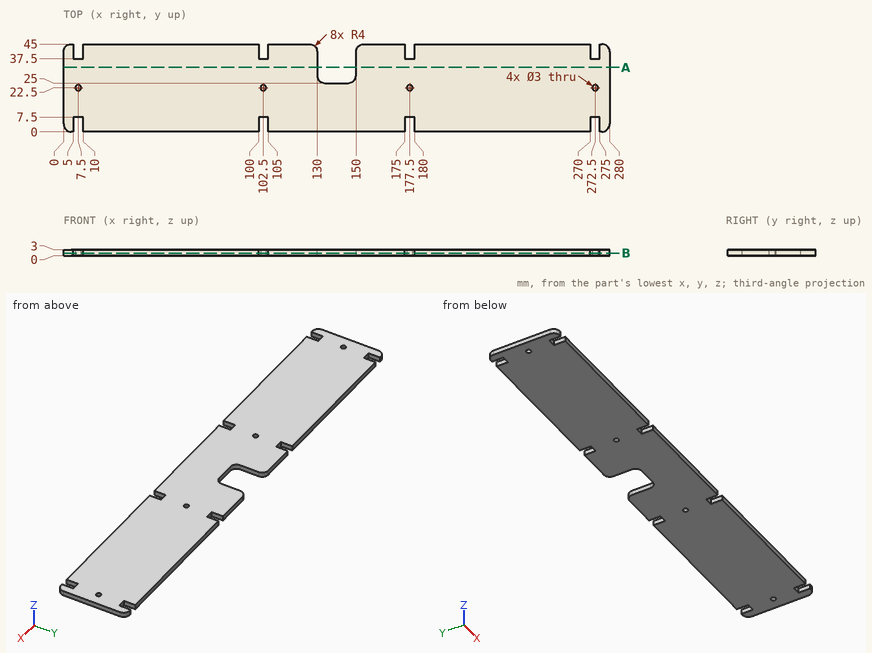
Could you check a few things on this drawing? It's one solid part, dimensions in mm from its lowest x, y, z. Give positions to 0.01 mm unless a question says otherwise; leave off trailing zeros. Loops run counter-clockwise (first coordinate to the right, second up) from the corner with the lowest first, then second, coordinate; pieces in that order, holes last. Notation, with made-up numbers: M 85,35.5 L 141,35.5 A30 cw 141,68.5 Z; hole C -22,-21 d8. An arc over 180 degrees is marked long. One line per question, with ' | ' between items. Start each with the question number.
Q1. If I drill on line 1 (X direction, y = 23.5, z = 0.95); line 2 (X direction, y = 37, z = 2.45); line 3 (Y direction, x = 177.5, z = 1.3), over which ranges is the centre line in solid material (lowest first)? Write a range as from..to.
Q2. If we section it at B-B (z = 1.25): State how many separate pieces and enclosed holes the cut face has, plus the area to 3 significant figures.
Q3. For pin 1 Ø0.9 at (y, z) = (41.5, 2) entering from -X; pin 2 Ø0.9 at (x, z) = (272, 2) entering from +Y; pin 3 Ø0.9 at (y, z) = (42.5, 1) entering from +X; pin 4 Ø0.9 at (x, z) = (103.5, 2) entering from -Y, each with a flat end and sliding along its axis, tell me the tip position at first contact or that it passes through.
Q4. If we section it at A-A (y = 33): Please give me the cut outline in (x, z), plus the area to 3 significant figures.
Computed:
1) line 1: x = 0..6.38, 8.62..101.38, 103.62..176.38, 178.62..271.38, 273.62..280 | line 2: x = 0..130, 150..280 | line 3: y = 7.5..21, 24..37.5
2) separate pieces: 1 | enclosed holes: 4 | area: 11,900 mm²
3) pin 1: stops at x = 0 | pin 2: stops at y = 37.5 | pin 3: stops at x = 279.86 | pin 4: stops at y = 7.5
4) outline: M 0,0 L 130,0 L 130,3 L 0,3 Z; M 150,0 L 280,0 L 280,3 L 150,3 Z | area: 780 mm²
